Can you work these out from the model? Positions are in its coordinate system, mm. Face numbers are marked on the shaded views. A direction names the side the tool comes from. Coordinates: 2 decimals unless noted, no trailing zeros. Order: outer loops, then holes, each group sorted by start corner. A loop starts at its lowest first (then second) coordinate and runs counter-clockwise, first axis right, second up. Notation, with made-up numbers: (-29, 88.5) -> (-7, 88.5) arc R38 cw to (-7, 127.5) -> close; hole circle Ø2 at (65, 52). An arc over 180 degrees is marked (long way). Write item = value, one per line.
```python
from build123d import *

# Parameters (mm, degrees)
F1_DEPTH = 3
F3_D     = 1
F5_D     = 1


with BuildPart() as f1:
    # F0 (on Top) → F1 (new body)
    with BuildSketch(Plane.XY):
        Polygon((6, 0), (0, 0), (0, -15), (34, -15), (34, 0), (28, 0), (28, -12), (6, -12), align=None)
    extrude(amount=F1_DEPTH)

    # F3 (through all)
    with Locations(Plane(origin=(0, 0, 0), x_dir=(1, 0, 0), z_dir=(0, 0, -1))):
        with Locations((4, 6)):
            Hole(F3_D / 2)

    # F5 (through all)
    with Locations(Plane(origin=(0, 0, 0), x_dir=(1, 0, 0), z_dir=(0, 0, -1))):
        with Locations((29.9340598285, 6)):
            Hole(F5_D / 2)


solid = f1.part
```
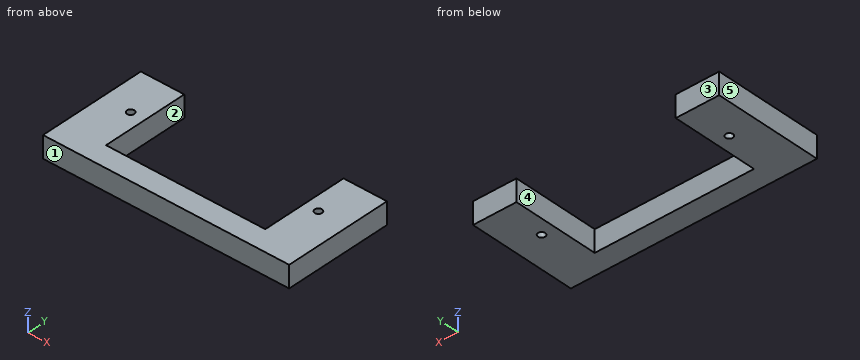
Item 1: I'm going to push a flat-ended pin straight in: P1, Ø1.5, axis at x = 14.5, z = 1.5, coming from the +Y side. Where does the tip first touch, or does it pass through?
A:
P1 = -12
Item 2: If we mould it in two halves opening along X, with no side actions, what happens to the marked faces 3, 4 and 5? For each: pulls with the +X half, pulls with the -X half, needs draft (parallel to the pull), parting line crosses it, or undercut.
A:
face_3 = needs draft
face_4 = undercut
face_5 = pulls with the -X half
Item 3: I want a section at B-B, the plane y = -0.75. Please give me the cut outline in (x, z), plus the area to 3 significant figures.
A:
outline = (0, 0) -> (6, 0) -> (6, 3) -> (0, 3) -> close; (28, 0) -> (34, 0) -> (34, 3) -> (28, 3) -> close
area = 36.0 mm2
Item 4: If I drill on probe 1 along X at (y, z) = (-6, 2.25); probe 2 along X at (y, z) = (-1.25, 1.95); probe 3 along Y at (x, z) = (4, 0.75), over which ranges is the centre line in solid material (lowest first)?
A:
probe_1 = 0 to 3.5, 4.5 to 6, 28 to 29.43, 30.43 to 34
probe_2 = 0 to 6, 28 to 34
probe_3 = -15 to -6.5, -5.5 to 0
Item 5: For the marked faces 1 and 2, which set-ups out of +Z, -Z, +X, -X, +Y, -Y let a thin tool reach every point of the face, with its end or its side?
A:
face_1 = +Z, -Z, +X, -X, -Y
face_2 = +Z, -Z, +Y
Item 6: I want a section at A-A, the plane x = 4. Please give me the cut outline in (y, z).
A:
outline = (-15, 0) -> (-6.5, 0) -> (-6.5, 3) -> (-15, 3) -> close; (-5.5, 0) -> (0, 0) -> (0, 3) -> (-5.5, 3) -> close
Item 7: I want a section at C-C, the plane y = -6. Please give me the cut outline in (x, z), plus the area to 3 significant figures.
A:
outline = (0, 0) -> (3.5, 0) -> (3.5, 3) -> (0, 3) -> close; (4.5, 0) -> (6, 0) -> (6, 3) -> (4.5, 3) -> close; (28, 0) -> (29.43, 0) -> (29.43, 3) -> (28, 3) -> close; (30.43, 0) -> (34, 0) -> (34, 3) -> (30.43, 3) -> close
area = 30.0 mm2
Item 8: I want a section at D-D, the plane z = 2.15. Please give me the cut outline in (x, y).
A:
outline = (0, -15) -> (34, -15) -> (34, 0) -> (28, 0) -> (28, -12) -> (6, -12) -> (6, 0) -> (0, 0) -> close; hole circle Ø1 at (4, -6); hole circle Ø1 at (29.93, -6)
